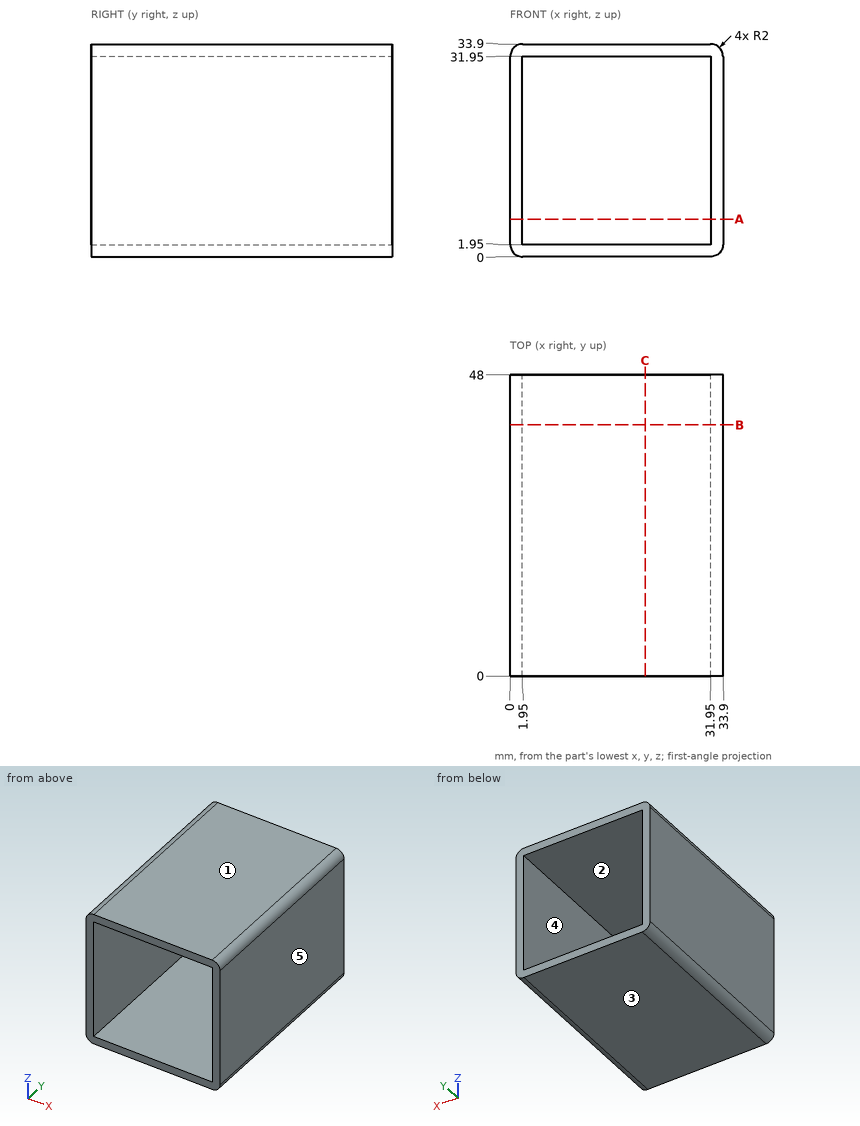
Can you work these out from the drawing? Everything is in mm from the part's minimum corner. A direction names the side the tool comes from. Coordinates: 2 decimals unless noted, no trailing zeros. Order: outer loops, then holes, each group sorted by start corner. A loop starts at its lowest first (then second) coordinate and runs counter-clockwise, first axis right, second up. Notation, with made-up numbers: (85.5, 54.5) -> (96.5, 54.5) arc R31 cw to (96.5, 79.5) -> close; hole circle Ø3 at (11, 60). An arc over 180 degrees is marked (long way). Return JSON: item names as keys, results as strings.
1) I'm going to push a flat-ended pin straight in: P1, Ø12, axis at y = 15, z = 4, coming from the -X side. Where does the tip first touch, or does it pass through?
Conclusion:
{"P1": "stops at x = 0"}
2) If we section it at C-C on x = 21.5: List the corners of the cut face in (y, z) for me.
Conclusion:
{"outline": "(0, 0) -> (48, 0) -> (48, 1.95) -> (0, 1.95) -> close; (0, 31.95) -> (48, 31.95) -> (48, 33.9) -> (0, 33.9) -> close"}
3) On a 3-axis mill with a long thin cutter (end or side, diameter ignored), from which of +Z, -Z, +X, -X, +Y, -Y can I reach the whole of each face in a straight line? I mean the marked faces 4 and 5. Say none if no direction works.
Conclusion:
{"face 4": "+Y, -Y", "face 5": "+Z, -Z, +X, +Y, -Y"}
4) Thinking about a two-plate mould opening in Z: for the marked faces 1, 2 and 3, which applies, +Z half, -Z half, draft (parallel to the pull), parting line (faces both ways), or undercut?
Conclusion:
{"face 1": "+Z half", "face 2": "undercut", "face 3": "-Z half"}
5) If we section it at A-A on z = 6: List the corners of the cut face in (x, y) for me, plus the area to 3 significant figures.
Conclusion:
{"outline": "(0, 0) -> (1.95, 0) -> (1.95, 48) -> (0, 48) -> close; (31.95, 0) -> (33.9, 0) -> (33.9, 48) -> (31.95, 48) -> close", "area": "187 mm²"}
6) If we section it at B-B on y = 40: List the corners of the cut face in (x, z) for me.
Conclusion:
{"outline": "(0, 2) arc R2 ccw to (2, 0) -> (31.9, 0) arc R2 ccw to (33.9, 2) -> (33.9, 31.9) arc R2 ccw to (31.9, 33.9) -> (2, 33.9) arc R2 ccw to (0, 31.9) -> close; hole (1.95, 1.95) -> (31.95, 1.95) -> (31.95, 31.95) -> (1.95, 31.95) -> close"}
7) If I drill on probe 1 along Z at (x, y) = (13, 37), over which ranges is the centre line in solid material (lowest first)?
Conclusion:
{"probe 1": "z = 0 to 1.95, 31.95 to 33.9"}
